Source: CAD feature listing. Evaluate the final solid. Frame: model axes, mm. Coordinates: 2 decimals unless noted, no trailing zeros. Order: outer loops, then holes, each group sorted by start corner. A loop starts at its lowest first (then second) coordinate and runs counter-clockwise, first axis right, second up.
```python
from build123d import *

# Parameters (mm, degrees)
SKETCH1_W           = 22.95
SKETCH1_H           = 22.95
SKETCH1_W_2         = 22.45
SKETCH1_H_2         = 22.45
SKETCH1_W_3         = 0.25
SKETCH1_H_3         = 9.5
SKETCH1_W_4         = 9.5
SKETCH1_H_4         = 0.25
SKETCH1_R           = 0.975
SKETCH1_H_5         = 1
SKETCH1_W_5         = 1
BOSS_EXTRUDE5_DEPTH = 0.2


with BuildPart() as part:
    # Sketch1 → Boss-Extrude5 (new body)
    # profile 1 of 26: a face of its own
    with BuildSketch(Plane(origin=(0, 0, 0), x_dir=(1, 0, 0), z_dir=(0, 1, 0))):
        Rectangle(SKETCH1_W, SKETCH1_H)
        Rectangle(SKETCH1_W_2, SKETCH1_H_2, mode=Mode.SUBTRACT)
    # profile 2 of 26: a face of its own
    with BuildSketch(Plane(origin=(0, 0, 0), x_dir=(1, 0, 0), z_dir=(0, 1, 0))):
        with Locations((-1.6, -6.475)):
            Rectangle(SKETCH1_W_3, SKETCH1_H_3)
    # profile 3 of 26: a face of its own
    with BuildSketch(Plane(origin=(0, 0, 0), x_dir=(1, 0, 0), z_dir=(0, 1, 0))):
        with Locations((-6.475, -1.6)):
            Rectangle(SKETCH1_W_4, SKETCH1_H_4)
    # profile 4 of 26: a face of its own
    with BuildSketch(Plane(origin=(0, 0, 0), x_dir=(1, 0, 0), z_dir=(0, 1, 0))):
        Polygon((-1.475, -1.475), (-1.475, -1.725), (1.475, -1.725), (1.475, -1.475), (1.725, -1.475), (1.725, 1.475), (1.475, 1.475), (1.475, 1.725), (-1.475, 1.725), (-1.475, 1.475), (-1.725, 1.475), (-1.725, -1.475), align=None)
        with Locations(Location((0, 0, 0), (0, 0, 270))):
            Circle(SKETCH1_R, mode=Mode.SUBTRACT)
    # profile 5 of 26: a face of its own
    with BuildSketch(Plane(origin=(0, 0, 0), x_dir=(1, 0, 0), z_dir=(0, 1, 0))):
        with Locations((-1.6, -1.6)):
            Rectangle(SKETCH1_W_3, SKETCH1_H_4)
    # profile 6 of 26: a face of its own
    with BuildSketch(Plane(origin=(0, 0, 0), x_dir=(1, 0, 0), z_dir=(0, 1, 0))):
        with Locations((1.6, -1.6)):
            Rectangle(SKETCH1_W_3, SKETCH1_H_4)
    # profile 7 of 26: a face of its own
    with BuildSketch(Plane(origin=(0, 0, 0), x_dir=(1, 0, 0), z_dir=(0, 1, 0))):
        with Locations((6.475, -1.6)):
            Rectangle(SKETCH1_W_4, SKETCH1_H_4)
    # profile 8 of 26: a face of its own
    with BuildSketch(Plane(origin=(0, 0, 0), x_dir=(1, 0, 0), z_dir=(0, 1, 0))):
        with Locations((1.6, -6.475)):
            Rectangle(SKETCH1_W_3, SKETCH1_H_3)
    # profile 9 of 26: a face of its own
    with BuildSketch(Plane(origin=(0, 0, 0), x_dir=(1, 0, 0), z_dir=(0, 1, 0))):
        with Locations((1.6, 1.6)):
            Rectangle(SKETCH1_W_3, SKETCH1_H_4)
    # profile 10 of 26: a face of its own
    with BuildSketch(Plane(origin=(0, 0, 0), x_dir=(1, 0, 0), z_dir=(0, 1, 0))):
        with Locations((6.475, 1.6)):
            Rectangle(SKETCH1_W_4, SKETCH1_H_4)
    # profile 11 of 26: a face of its own
    with BuildSketch(Plane(origin=(0, 0, 0), x_dir=(1, 0, 0), z_dir=(0, 1, 0))):
        with Locations((1.6, 6.475)):
            Rectangle(SKETCH1_W_3, SKETCH1_H_3)
    # profile 12 of 26: a face of its own
    with BuildSketch(Plane(origin=(0, 0, 0), x_dir=(1, 0, 0), z_dir=(0, 1, 0))):
        with Locations((-1.6, 1.6)):
            Rectangle(SKETCH1_W_3, SKETCH1_H_4)
    # profile 13 of 26: a face of its own
    with BuildSketch(Plane(origin=(0, 0, 0), x_dir=(1, 0, 0), z_dir=(0, 1, 0))):
        with Locations((-6.475, 1.6)):
            Rectangle(SKETCH1_W_4, SKETCH1_H_4)
    # profile 14 of 26: a face of its own
    with BuildSketch(Plane(origin=(0, 0, 0), x_dir=(1, 0, 0), z_dir=(0, 1, 0))):
        with Locations((-1.6, 6.475)):
            Rectangle(SKETCH1_W_3, SKETCH1_H_3)
    # profile 15 of 26: a face of its own
    with BuildSketch(Plane(origin=(0, 0, 0), x_dir=(1, 0, 0), z_dir=(0, 1, 0))):
        with Locations((-11.6, -1.95)):
            Rectangle(SKETCH1_W_3, SKETCH1_H_5)
    # profile 16 of 26: a face of its own
    with BuildSketch(Plane(origin=(0, 0, 0), x_dir=(1, 0, 0), z_dir=(0, 1, 0))):
        with Locations((-11.6, 1.95)):
            Rectangle(SKETCH1_W_3, SKETCH1_H_5)
    # profile 17 of 26: a face of its own
    with BuildSketch(Plane(origin=(0, 0, 0), x_dir=(1, 0, 0), z_dir=(0, 1, 0))):
        with Locations((11.6, -1.95)):
            Rectangle(SKETCH1_W_3, SKETCH1_H_5)
    # profile 18 of 26: a face of its own
    with BuildSketch(Plane(origin=(0, 0, 0), x_dir=(1, 0, 0), z_dir=(0, 1, 0))):
        with Locations((11.6, 1.95)):
            Rectangle(SKETCH1_W_3, SKETCH1_H_5)
    # profile 19 of 26: a face of its own
    with BuildSketch(Plane(origin=(0, 0, 0), x_dir=(1, 0, 0), z_dir=(0, 1, 0))):
        with Locations((1.95, -11.6)):
            Rectangle(SKETCH1_W_5, SKETCH1_H_4)
    # profile 20 of 26: a face of its own
    with BuildSketch(Plane(origin=(0, 0, 0), x_dir=(1, 0, 0), z_dir=(0, 1, 0))):
        with Locations((-1.95, -11.6)):
            Rectangle(SKETCH1_W_5, SKETCH1_H_4)
    # profile 21 of 26: a face of its own
    with BuildSketch(Plane(origin=(0, 0, 0), x_dir=(1, 0, 0), z_dir=(0, 1, 0))):
        with Locations((1.95, 11.6)):
            Rectangle(SKETCH1_W_5, SKETCH1_H_4)
    # profile 22 of 26: a face of its own
    with BuildSketch(Plane(origin=(0, 0, 0), x_dir=(1, 0, 0), z_dir=(0, 1, 0))):
        with Locations((-1.95, 11.6)):
            Rectangle(SKETCH1_W_5, SKETCH1_H_4)
    # profile 23 of 26: a face of its own
    with BuildSketch(Plane(origin=(0, 0, 0), x_dir=(1, 0, 0), z_dir=(0, 1, 0))):
        Polygon((-11.975, -2.45), (-11.725, -2.45), (-11.725, -1.45), (-11.725, 1.45), (-11.725, 2.45), (-11.975, 2.45), align=None)
    # profile 24 of 26: a face of its own
    with BuildSketch(Plane(origin=(0, 0, 0), x_dir=(1, 0, 0), z_dir=(0, 1, 0))):
        Polygon((2.45, -11.975), (2.45, -11.725), (1.45, -11.725), (-1.45, -11.725), (-2.45, -11.725), (-2.45, -11.975), align=None)
    # profile 25 of 26: a face of its own
    with BuildSketch(Plane(origin=(0, 0, 0), x_dir=(1, 0, 0), z_dir=(0, 1, 0))):
        Polygon((11.725, -1.45), (11.725, -2.45), (11.975, -2.45), (11.975, 2.45), (11.725, 2.45), (11.725, 1.45), align=None)
    # profile 26 of 26: a face of its own
    with BuildSketch(Plane(origin=(0, 0, 0), x_dir=(1, 0, 0), z_dir=(0, 1, 0))):
        Polygon((1.45, 11.725), (2.45, 11.725), (2.45, 11.975), (-2.45, 11.975), (-2.45, 11.725), (-1.45, 11.725), align=None)
    extrude(amount=BOSS_EXTRUDE5_DEPTH)


solid = part.part
```
Q1. Section query D-D on z = 0. Output: boundary loops of the cut face in (x, y) (3 decimals).
Solutions:
outline: (-11.975, 0) - (-11.725, 0) - (-11.725, 0.2) - (-11.975, 0.2) - close; (-11.475, 0) - (-11.225, 0) - (-11.225, 0.2) - (-11.475, 0.2) - close; (-1.725, 0) - (-0.975, 0) - (-0.975, 0.2) - (-1.725, 0.2) - close; (0.975, 0) - (1.725, 0) - (1.725, 0.2) - (0.975, 0.2) - close; (11.225, 0) - (11.475, 0) - (11.475, 0.2) - (11.225, 0.2) - close; (11.725, 0) - (11.975, 0) - (11.975, 0.2) - (11.725, 0.2) - close
Q2. Pin query (flat end, axial travel): P1, Ø1.5, axis at x = 7.5, z = 4, coming from the +Y side. Return the tip coordinate at first contact, or that it passes through.
Solutions:
P1: passes through
Q3. Section query B-B on z = 10.75. Output: boundary loops of the cut face in (x, y) (3 decimals), plus the area to 3 significant figures.
Solutions:
outline: (-11.475, 0) - (-11.225, 0) - (-11.225, 0.2) - (-11.475, 0.2) - close; (-1.725, 0) - (-1.475, 0) - (-1.475, 0.2) - (-1.725, 0.2) - close; (1.475, 0) - (1.725, 0) - (1.725, 0.2) - (1.475, 0.2) - close; (11.225, 0) - (11.475, 0) - (11.475, 0.2) - (11.225, 0.2) - close
area: 0.200 mm2
Q4. Material intervals for line 1 along X through (y, z) = (0.1, 0) (3 decimals); line 2 along Z through (x, y) = (-9, 0.15) (3 decimals), sorted ascending.
Solutions:
line 1: x = -11.975 to -11.725, -11.475 to -11.225, -1.725 to -0.975, 0.975 to 1.725, 11.225 to 11.475, 11.725 to 11.975
line 2: z = -11.475 to -11.225, -1.725 to -1.475, 1.475 to 1.725, 11.225 to 11.475
Q5. Section query A-A on x = 6.75. Output: boundary loops of the cut face in (y, z) (3 decimals).
Solutions:
outline: (0, -11.475) - (0.2, -11.475) - (0.2, -11.225) - (0, -11.225) - close; (0, -1.725) - (0.2, -1.725) - (0.2, -1.475) - (0, -1.475) - close; (0, 1.475) - (0.2, 1.475) - (0.2, 1.725) - (0, 1.725) - close; (0, 11.225) - (0.2, 11.225) - (0.2, 11.475) - (0, 11.475) - close
Q6. Section query C-C on x = 0. Output: boundary loops of the cut face in (y, z) (3 decimals), plus the area to 3 significant figures.
Solutions:
outline: (0, -11.975) - (0.2, -11.975) - (0.2, -11.725) - (0, -11.725) - close; (0, -11.475) - (0.2, -11.475) - (0.2, -11.225) - (0, -11.225) - close; (0, -1.725) - (0.2, -1.725) - (0.2, -0.975) - (0, -0.975) - close; (0, 0.975) - (0.2, 0.975) - (0.2, 1.725) - (0, 1.725) - close; (0, 11.225) - (0.2, 11.225) - (0.2, 11.475) - (0, 11.475) - close; (0, 11.725) - (0.2, 11.725) - (0.2, 11.975) - (0, 11.975) - close
area: 0.500 mm2
